Read the model definition and answer for the solid it produces. Units are mm, in the model's axes. Face numbers are marked on the shaded views. Coordinates: 2 decimals unless noted, no trailing zeros. Loops run counter-clockwise (first coordinate to the right, second up) from the corner with the lowest first, then second, coordinate; pieces in that order, holes last. Notation, with made-up numbers: (12, -32) -> (55, -32) arc R29 cw to (55, -9) -> close; hole circle Ø9 at (-37, 35.5). An arc over 180 degrees is marked (long way). Answer in a Markdown table with one row per item.
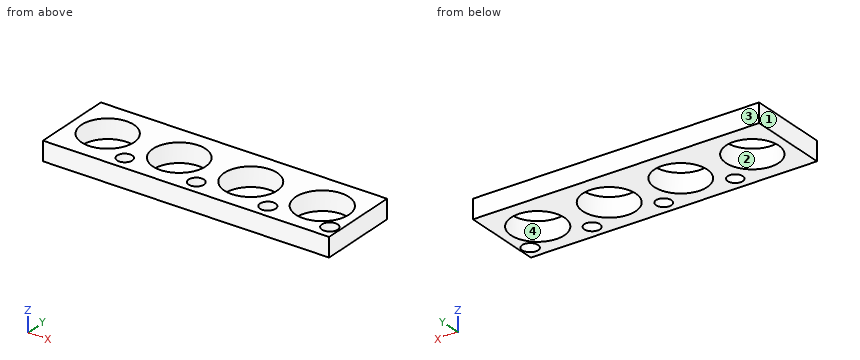
```python
from build123d import *

# Parameters (mm, degrees)
COUPON_PLATE_PROFILE_W                     = 120
COUPON_PLATE_PROFILE_H                     = 34
COUPON_PLATE_DEPTH                         = 8
BEARING_FIT_TRIAL_THROUGH_START            = -1
BEARING_SEAT_TRIAL_22P0_22P1_22P2_22P3_R   = 11
BEARING_SEAT_TRIAL_22P0_22P1_22P2_22P3_R_2 = 11.05
BEARING_SEAT_TRIAL_22P0_22P1_22P2_22P3_R_3 = 11.1
BEARING_SEAT_TRIAL_22P0_22P1_22P2_22P3_R_4 = 11.15
BEARING_FIT_TRIAL_THROUGH_DEPTH            = 64.872887638
DOWEL_FIT_TRIAL_THROUGH_START              = -1
DOWEL_TRIAL_6P35_6P45_6P55_6P65_R          = 3.175
DOWEL_TRIAL_6P35_6P45_6P55_6P65_R_2        = 3.225
DOWEL_TRIAL_6P35_6P45_6P55_6P65_R_3        = 3.275
DOWEL_TRIAL_6P35_6P45_6P55_6P65_R_4        = 3.325
DOWEL_FIT_TRIAL_THROUGH_DEPTH              = 64.872887638


with BuildPart() as part:
    # Coupon_plate_profile → Coupon_plate (new body)
    with BuildSketch(Plane.XY):
        Rectangle(COUPON_PLATE_PROFILE_W, COUPON_PLATE_PROFILE_H)
    extrude(amount=COUPON_PLATE_DEPTH)

    # Bearing_seat_trial_22p0_22p1_22p2_22p3 → Bearing_fit_trial_through (cut, through all)
    with BuildSketch(Plane.XY.offset(BEARING_FIT_TRIAL_THROUGH_START)):
        with Locations(Location((-45, 0, 0), (0, 0, 180))):
            Circle(BEARING_SEAT_TRIAL_22P0_22P1_22P2_22P3_R)
        with Locations(Location((-15, 0, 0), (0, 0, 180))):
            Circle(BEARING_SEAT_TRIAL_22P0_22P1_22P2_22P3_R_2)
        with Locations(Location((15, 0, 0), (0, 0, 180))):
            Circle(BEARING_SEAT_TRIAL_22P0_22P1_22P2_22P3_R_3)
        with Locations(Location((45, 0, 0), (0, 0, 180))):
            Circle(BEARING_SEAT_TRIAL_22P0_22P1_22P2_22P3_R_4)
    extrude(amount=BEARING_FIT_TRIAL_THROUGH_DEPTH, mode=Mode.SUBTRACT)

    # Dowel_trial_6p35_6p45_6p55_6p65 → Dowel_fit_trial_through (cut, through all)
    with BuildSketch(Plane.XY.offset(DOWEL_FIT_TRIAL_THROUGH_START)):
        with Locations(Location((-30, -11, 0), (0, 0, 180))):
            Circle(DOWEL_TRIAL_6P35_6P45_6P55_6P65_R)
        with Locations(Location((0, -11, 0), (0, 0, 180))):
            Circle(DOWEL_TRIAL_6P35_6P45_6P55_6P65_R_2)
        with Locations(Location((30, -11, 0), (0, 0, 180))):
            Circle(DOWEL_TRIAL_6P35_6P45_6P55_6P65_R_3)
        with Locations(Location((56, -11, 0), (0, 0, 180))):
            Circle(DOWEL_TRIAL_6P35_6P45_6P55_6P65_R_4)
    extrude(amount=DOWEL_FIT_TRIAL_THROUGH_DEPTH, mode=Mode.SUBTRACT)


solid = part.part
```
1. A cutting plane is placed at D-D on x = 15. Give the vertices of the cut face in (y, z), and give its area (3 significant figures).
A:
| item | result |
|---|---|
| outline | (-17, 0) -> (-11.1, 0) -> (-11.1, 8) -> (-17, 8) -> close; (11.1, 0) -> (17, 0) -> (17, 8) -> (11.1, 8) -> close |
| area | 94.4 mm2 |
2. Given pin 1 Ø13.5 at (x, y) = (-15, 0) entering from -Z; pin 2 Ø8 at (x, y) = (-43, -8) entering from +Z, each flat-ended and moving along its own axis, determine where each tip first touches the part or whether it passes through.
A:
| item | result |
|---|---|
| pin 1 | passes through |
| pin 2 | stops at z = 8 |
3. A cutting plane is placed at A-A on x = 0. Give the vertices of the cut face in (y, z) (3 decimals).
A:
| item | result |
|---|---|
| outline | (-17, 0) -> (-14.225, 0) -> (-14.225, 8) -> (-17, 8) -> close; (-7.775, 0) -> (17, 0) -> (17, 8) -> (-7.775, 8) -> close |
4. The mould has two halves that part along Y. Classify the marked faces 1, 2, 3 and 4: pulls with the +Y half, pulls with the -Y half, needs draft (parallel to the pull), parting line crosses it, or undercut.
A:
| item | result |
|---|---|
| face 1 | needs draft |
| face 2 | undercut |
| face 3 | pulls with the +Y half |
| face 4 | undercut |
5. A cutting plane is placed at B-B on y = 0. Give the vertices of the cut face in (x, z), and give its area (3 significant figures).
A:
| item | result |
|---|---|
| outline | (-60, 0) -> (-56, 0) -> (-56, 8) -> (-60, 8) -> close; (-34, 0) -> (-26.05, 0) -> (-26.05, 8) -> (-34, 8) -> close; (-3.95, 0) -> (3.9, 0) -> (3.9, 8) -> (-3.95, 8) -> close; (26.1, 0) -> (33.85, 0) -> (33.85, 8) -> (26.1, 8) -> close; (56.15, 0) -> (60, 0) -> (60, 8) -> (56.15, 8) -> close |
| area | 251 mm2 |
6. Find the intervals of material crossed by probe 1 along Y at (x, z) = (0, 1.25) (3 decimals); probe 2 along Y at (x, z) = (46, 3); probe 3 along X at (y, z) = (4, 2.5), in increasing order.
A:
| item | result |
|---|---|
| probe 1 | y = -17 to -14.225, -7.775 to 17 |
| probe 2 | y = -17 to -11.11, 11.11 to 17 |
| probe 3 | x = -60 to -55.25, -34.75 to -25.3, -4.7 to 4.65, 25.35 to 34.59, 55.41 to 60 |
7. A cutting plane is placed at C-C on z = 2.75. Count the separate pieces of the cut face and the enclosed holes in it, and give its area (3 significant figures).
A:
| item | result |
|---|---|
| separate pieces | 1 |
| enclosed holes | 8 |
| area | 2,410 mm2 |
